Could you check a few things on this model? Use its own coordinates, in mm. A direction names the side the tool comes from. Coordinates: 2 decimals unless noted, no trailing zeros.
1) Will these pins go through, and if not, where does the flat tip stop? P1, Ø8, axis at x = 1, z = 7.5, coming from the -Y side; P2, Ø2, axis at x = -12, z = 13.5, coming from the -Y side.
2) For faces 1 (the face through (-13.21, -79.75, 24.49)), 2 (the face through (-0.645, 27, 13)), 3 (the face through (-15.853, 56, 10)), 4 (the face through (-13.74, -79.75, 5.44)), 5 (the face through (-31.617, -11.482, 0.955)), which set-ups out of +Z, -Z, +X, -X, +Y, -Y let a thin tool reach every point of the face, with its end or its side?
3) Imagine slicing it at A-A on x = -2. Give the number of separate pieces and of enclosed holes in the cut face, plus the area to 3 significant figures.
4) If I drill on line 1 along Y through (x, z) = (-17, 4); line 2 along Y through (x, z) = (1, 12.7); line 3 along Y through (x, z) = (-4.5, 15), over which ranges is the centre line in solid material (lowest first)?
5) Thinking about a two-plate mould opening in X: for faces 6 (the face through (-3.52, 41.69, 12.52)), 7 (the face through (-31.617, -11.482, 24.445)), 8 (the face through (-4, 59, 13)), which applies, released by +X, released by -X, zero draft, split by the parting line, or undercut?
```python
from build123d import *

# Parameters (mm, degrees)
F0_W      = 38.1
F0_H      = 139.7
F0_R      = 12.827
F1_DEPTH  = 25.4
F3_DEPTH  = 25.4
F4_R      = 4.7625
F5_DEPTH  = 127
F6_R      = 6.35
F7_DEPTH  = 50.8
F8_W      = 23.3431950331
F8_H      = 12.7
F9_DEPTH  = 76.2
F10_R     = 3.17499
F12_DEPTH = 25.4


# Not quite as in the source:
# - a fillet or chamfer is up to 0.001 mm smaller than in the source, because OpenCascade refuses the exact size


with BuildPart() as f1:
    # F0 (on Top) → F1 (new body)
    with BuildSketch(Plane.XY):
        with Locations((-13.4720488012, -10.8498208284)):
            Rectangle(F0_W, F0_H)
        with Locations((-13.4720488012, 33.6001791716)):
            Circle(F0_R, mode=Mode.SUBTRACT)
    extrude(amount=F1_DEPTH)

    # F2 (on face) → F3 (cut)
    with BuildSketch(Plane.XY.offset(25.4)):
        with BuildLine():
            Line((-11.0907988012, 46.2042093777), (-11.0907988012, 59.0001791716))
            Line((-11.0907988012, 59.0001791716), (-15.8532988012, 59.0001791716))
            Line((-15.8532988012, 59.0001791716), (-15.8532988012, 46.2042093777))
            ThreePointArc((-15.8532988012, 46.2042093777), (-13.4720488012, 46.4271791716), (-11.0907988012, 46.2042093777))
        make_face()
    extrude(amount=-F3_DEPTH, mode=Mode.SUBTRACT)

    # F4 (on face) → F5 (cut)
    with BuildSketch(Plane(origin=(-32.5220488012, 0, 0), x_dir=(0, -1, 0), z_dir=(-1, 0, 0))):
        with Locations((-50.9158676147, 12.7)):
            Circle(F4_R)
    extrude(amount=-F5_DEPTH, mode=Mode.SUBTRACT)

    # F6 (on face) → F7 (cut)
    with BuildSketch(Plane.XY.offset(25.4)):
        with Locations((-13.4720488012, -63.2373208284)):
            Circle(F6_R)
    extrude(amount=-F7_DEPTH, mode=Mode.SUBTRACT)

    # F8 (on face) → F9 (cut)
    with BuildSketch(Plane.YZ.offset(5.5779511988)):
        with Locations((-69.0282233119, 12.7)):
            Rectangle(F8_W, F8_H)
        with BuildLine():
            Line((-57.3566257954, 19.05), (-57.3566257954, 6.35))
            ThreePointArc((-57.3566257954, 6.35), (-51.0066257954, 12.7), (-57.3566257954, 19.05))
        make_face()
    extrude(amount=-F9_DEPTH, mode=Mode.SUBTRACT)

    # F10 (radius 3.175 in the source; OpenCascade refuses exactly that, so slightly less here)
    f10_edges = [f1.edges().sort_by_distance(p)[0] for p in [
        (5.577951, -69.028223, 19.05),
        (-13.472049, -80.699821, 6.35),
        (5.577951, -10.849821, 25.4),
        (-32.522049, -10.849821, 25.4),
        (-13.472049, -80.699821, 25.4),
        (5.577951, -10.849821, 0),
        (-13.472049, -80.699821, 0),
        (-24.187674, 59.000179, 25.4),
        (-2.756424, 59.000179, 25.4),
        (-32.522049, 59.000179, 12.7),
        (5.577951, 59.000179, 12.7),
        (-2.756424, 59.000179, 0),
        (-24.187674, 59.000179, 0),
        (-32.522049, -10.849821, 0),
        (-13.472049, -80.699821, 19.05),
        (-32.522049, -51.006626, 12.7),
        (-32.522049, -69.028223, 6.35),
        (-32.522049, -69.028223, 19.05),
    ]]
    fillet(f10_edges, radius=F10_R)

    # F11 (on face) → F12 (cut)
    with BuildSketch(Plane.XY.offset(25.4)):
        with BuildLine():
            Line((-0.6450488012, 20.9001791716), (-0.6450488012, 33.6001791716))
            ThreePointArc((-0.6450488012, 33.6001791716), (-4.3126364935, 24.6203631836), (-13.2180736983, 20.7756937765))
            Line((-13.2180736983, 20.7756937765), (-0.6450488012, 20.9001791716))
        make_face()
    extrude(amount=-F12_DEPTH, mode=Mode.SUBTRACT)


solid = f1.part
```
Filled in:
1. P1: stops at y = -80.68
1. P2: stops at y = -51.27
2. face 1: +Z, +X, -X, -Y
2. face 2: +Z, -Z
2. face 3: +Z, -Z, +Y
2. face 4: +X, -X, -Y
2. face 5: -Z, -X, +Y, -Y
3. separate pieces: 2
3. enclosed holes: 1
3. area: 2,640 mm2
4. line 1: y = -80.59 to -68.52, -57.96 to 21.27, 45.93 to 59
4. line 2: y = -51.01 to 46.15, 55.68 to 59
4. line 3: y = -51.44 to 20.86, 42.77 to 46.75, 55.09 to 59
5. face 6: undercut
5. face 7: released by -X
5. face 8: zero draft
